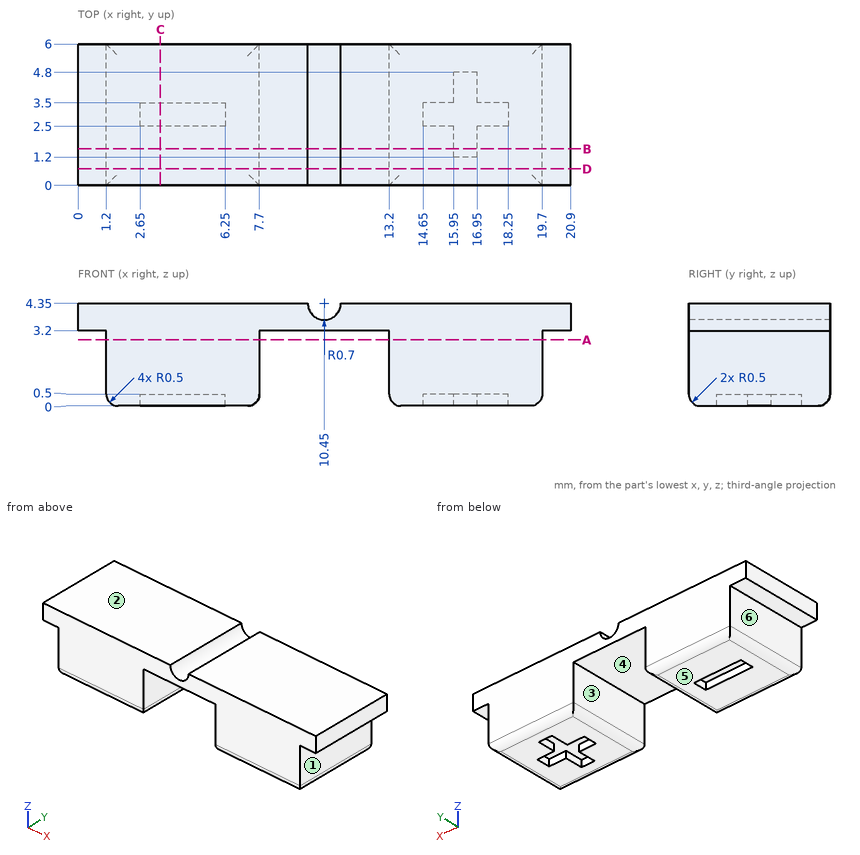
Design review of the part shown in the three views and the two pictorial views. Dimensions are in mm from the part's minimum x, y and z. A direction names the side the tool comes from. Give positions to 0.01 mm unless a question says otherwise; leave off trailing zeros. Write each loop counter-clockwise with the first axis right and the second up, starting at its lowest first coordinate (ties: lowest second). Pieces come first, ordered by that corner, then holes. Notation, with made-up numbers: M 57.25,46.25 L 92.25,46.25 A14 cw 92.25,55.25 Z; hole C 70.25,2.5 d5. An arc over 180 degrees is marked long. One line per question, with ' | ' between items. Start each with the question number.
Item 1: Wall thickness on line 1 (X direction, y = 4, z = 1.95); line 2 (X direction, y = 2.8, z = 0.35); line 3 (Z direction, x = 12.5, y = 5.2): over which ranges is each line inside the solid? List them lowest first. Write a range as from..to.
Item 2: For pin 1 (0.8 mm diameter, centred on x = 4.5, y = 3, fed in from -Z); pin 2 (1.3 mm diameter, centred on x = 0.5, y = 4, fed in from -Z); pin 3 (1.4 mm diameter, centred on y = 1.5, z = 2, fed in from +X), all flat-tipped, find the tip position at first contact; note any pin that passes through.
Item 3: We need section D-D on y = 0.7. Write out the cut boundary in (x, z), plus the area to 3 significant figures.
Item 4: We need section A-A on z = 2.8. Write out the cut boundary in (x, y), plus the area to 3 significant figures.
Item 5: We need section C-C on x = 3.5. Write out the cut boundary in (y, z).
Item 6: For the marked faces 1, 2 and 3, list the 3-axis set-ups (+Z, -Z, +X, -X, +Y, -Y) from which the entire face can be reached by the end or side of a thin tool; tool diameter is ignored.
Item 7: Draft analysis for pull direction X (two halves, no side actions). For the marked faces 4, 5 and 6, state which applies: released by +X, released by -X, zero draft, split by the parting line, or undercut.
Item 8: We need section B-B on y = 1.55. Write out the cut boundary in (x, z), plus the area to 3 significant figures.
Results found:
1) line 1: x = 1.2..7.7, 13.2..19.7 | line 2: x = 1.22..2.65, 6.25..7.68, 13.22..14.65, 18.25..19.68 | line 3: z = 3.2..4.35
2) pin 1: stops at z = 0.5 | pin 2: stops at z = 3.2 | pin 3: stops at x = 19.7
3) outline: M 0,3.2 L 1.2,3.2 L 1.2,0.5 A0.5 ccw 1.7,0 L 7.2,0 A0.5 ccw 7.7,0.5 L 7.7,3.2 L 13.2,3.2 L 13.2,0.5 A0.5 ccw 13.7,0 L 19.2,0 A0.5 ccw 19.7,0.5 L 19.7,3.2 L 20.9,3.2 L 20.9,4.35 L 11.15,4.35 A0.7 cw 9.75,4.35 L 0,4.35 Z | area: 64.7 mm2
4) outline: M 1.2,0 L 7.7,0 L 7.7,6 L 1.2,6 Z; M 13.2,0 L 19.7,0 L 19.7,6 L 13.2,6 Z | area: 78.0 mm2
5) outline: M 0,0.5 A0.5 ccw 0.5,0 L 2.5,0 L 2.5,0.5 L 3.5,0.5 L 3.5,0 L 5.5,0 A0.5 ccw 6,0.5 L 6,4.35 L 0,4.35 Z
6) face 1: -Z, +X, +Y, -Y | face 2: +Z, +X, -X, +Y, -Y | face 3: -Z, +Y, -Y
7) face 4: undercut | face 5: zero draft | face 6: released by -X
8) outline: M 0,3.2 L 1.2,3.2 L 1.2,0.5 A0.5 ccw 1.7,0 L 7.2,0 A0.5 ccw 7.7,0.5 L 7.7,3.2 L 13.2,3.2 L 13.2,0.5 A0.5 ccw 13.7,0 L 15.95,0 L 15.95,0.5 L 16.95,0.5 L 16.95,0 L 19.2,0 A0.5 ccw 19.7,0.5 L 19.7,3.2 L 20.9,3.2 L 20.9,4.35 L 11.15,4.35 A0.7 cw 9.75,4.35 L 0,4.35 Z | area: 64.2 mm2
